```python
from build123d import *

# Parameters (mm, degrees)
F0_W     = 3.1
F0_H     = 29.1
F0_W_2   = 3.1796320426
F0_H_2   = 29.3082972342
F2_R     = 5.95
F3_DEPTH = 25


with BuildPart() as f1:
    # F0 (on Front) → F1 (revolve)
    with BuildSketch(Plane.XZ):
        with Locations((1.55, 14.55)):
            Rectangle(F0_W, F0_H)
        Polygon((3.1, 29.1), (3.1, 0), (6.9484059341, 0), (6.9484059341, 19.0335457699), align=None)
        Polygon((6.9484059341, 19.0335457699), (6.9484059341, 0), (12.497687584, 0), (12.497687584, 19.122838374), align=None)
        Polygon((12.497687584, 19.122838374), (12.497687584, 0), (16.0203679574, 0), (16.0203679574, 29.3082972342), align=None)
        with Locations((17.6101839787, 14.6541486171)):
            Rectangle(F0_W_2, F0_H_2)
    revolve(axis=Axis((9.6, 0, 0), (1, 0, 0)))

    # F2 (on Right) → F3 (cut)
    with BuildSketch(Plane.YZ):
        Circle(F2_R)
    extrude(amount=F3_DEPTH, mode=Mode.SUBTRACT)


solid = f1.part
```
Build history of the part. All positions in model axes, mm. A direction names the side the tool comes from. Give positions to 0.01 mm unless a question says otherwise; leave off trailing zeros. Order: outer loops, then holes, each group sorted by start corner. A loop starts at its lowest first (then second) coordinate and runs counter-clockwise, first axis right, second up. Notation, with made-up numbers: M 75.25,4.5 L 124.25,4.5 A36 ccw 124.25,39.5 Z; hole C 17,1 d3. An arc over 180 degrees is marked long. Write item = value, one per line. Start each with the question number.
(1) Slice it at A-A on x = 8. Write the cut outline in (y, z).
(2) Probe L1, parallel to Y at x = 12, z = 0; L2, parallel to Y at x = 7.75, z = 3; L3, parallel to X at y = 4.5, z = -23. List the from-to ranges inside material, lowest first. Write a range as [from, to].
(3) Which spindle directions (+Z, -Z, +X, -X, +Y, -Y) get a long thin tool onto all of the face, cutting with end or side? Do faces 1 (the conical face through (12.67, 19.15, -4.25)), 2 (the cylindrical face through (9.466, -4.385, 4.021)), 3 (the cylindrical face through (1.572, -28.852, -3.788)). Say none if no direction does.
(4) Two-plate mould, pull along X, no slides. Class faces 4 (the conical face through (6.708, -5.906, 18.755)), 5 (the flat face through (19.2, 6.1, 0.4)), 6 (the conical face through (9.684, -18.915, -2.484)), 7 (the flat face through (0, 6.1, 0.4)): released by +X, released by -X, zero draft, split by the parting line, or undercut.
(5) Pin check, flat tips, straight feed: pin 1 Ø3 at (x, z) = (15, -0.5) entering from +Y; pin 2 Ø2 at (y, z) = (18.5, -2) entering from -X; pin 3 Ø9.5 at (y, z) = (0, 0) entering from -X; pin 4 Ø2 at (x, y) = (11.5, 2.5) entering from +Z. Stop position of each tip, or through.
(6) Slice it at B-B on x = 1.5. Write the cut outline in (y, z).
Responses:
q1.outline = C 0,0 d38.1; hole C 0,0 d11.9
q2.L1 = [-19.11, -5.95], [5.95, 19.11]
q2.L2 = [-18.81, -5.14], [5.14, 18.81]
q2.L3 = [0, 5.27], [13.99, 19.2]
q3.face_1 = none
q3.face_2 = +X, -X
q3.face_3 = -X
q4.face_4 = undercut
q4.face_5 = released by +X
q4.face_6 = undercut
q4.face_7 = released by -X
q5.pin_1 = 29.31
q5.pin_2 = 0
q5.pin_3 = through
q5.pin_4 = 19.05
q6.outline = C 0,0 d58.2; hole C 0,0 d11.9
